Verification items for this drawing (mm, ordinates from the low corner). A direction names the side the tool comes from. Coordinates: 2 decimals unless noted, no trailing zeros. Order: outer loops, then holes, each group sorted by start corner. A loop starts at its lowest first (then second) coordinate and runs counter-clockwise, first axis right, second up.
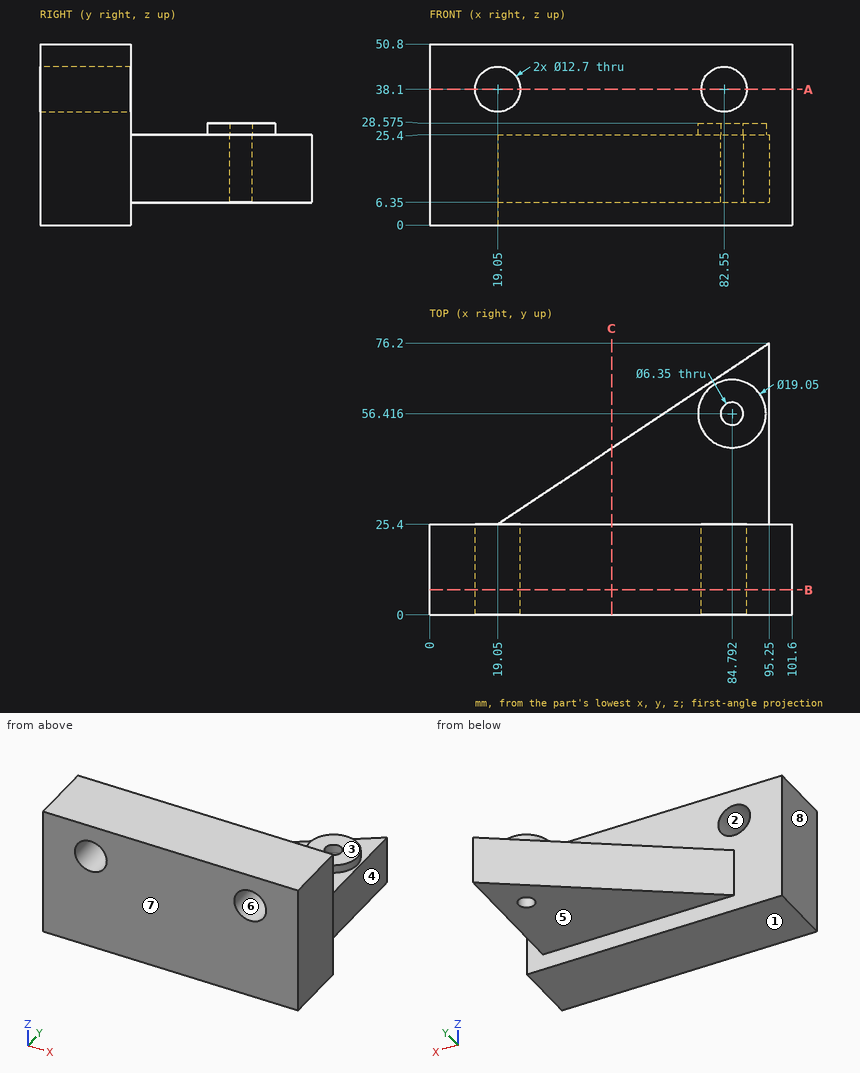
(1) Cross-section at B-B (y = 7). Enter the section's corners in (x, z), and give its area (3 significant figures).
Filled in:
outline: (0, 0) - (101.6, 0) - (101.6, 50.8) - (0, 50.8) - close; hole circle Ø12.7 at (19.05, 38.1); hole circle Ø12.7 at (82.55, 38.1)
area: 4,910 mm2
(2) Cross-section at A-A (z = 38.1). Enter the section's corners in (x, y).
Filled in:
outline: (0, 0) - (12.7, 0) - (12.7, 25.4) - (0, 25.4) - close; (25.4, 0) - (76.2, 0) - (76.2, 25.4) - (25.4, 25.4) - close; (88.9, 0) - (101.6, 0) - (101.6, 25.4) - (88.9, 25.4) - close
(3) Cross-section at C-C (x = 51). Enter the section's corners in (y, z).
Filled in:
outline: (0, 0) - (25.4, 0) - (25.4, 6.35) - (46.7, 6.35) - (46.7, 25.4) - (25.4, 25.4) - (25.4, 50.8) - (0, 50.8) - close
(4) Go/stop test with flat-tipped pins: P1, Ø2, axis at x = 31, z = 30.5, coming from the +Y side; P2, Ø8.5, axis at x = 84.79, y = 56.42, coming from the +Z side (3 decimals); P3, Ø15, axis at x = 67, y = 54.5, coming from the +Z side. Record where each tip stops, or that it passes through.
Filled in:
P1: stops at y = 25.4
P2: stops at z = 28.575
P3: stops at z = 25.4
(5) Tool access check on the marked faces 1, 2, 3, 4 and 5. Record the directions out of +Z, -Z, +X, -X, +Y, -Y that give a thin tool (end or side, any length) a straight path to the whole face; none if there is none.
Filled in:
face 1: -Z, +X, -X, +Y, -Y
face 2: +Y, -Y
face 3: +Z, +X, -X, +Y
face 4: +Z, -Z, +X, +Y
face 5: -Z, +X, -X, +Y
(6) Release check for a two-part mould opening along X. For the marked faces 6, 7 and 8 record: +X half, -X half, draft (parallel to the pull), parting line (faces both ways), or undercut.
Filled in:
face 6: undercut
face 7: draft
face 8: -X half
(7) Thickness scan on probe 1 along X at (y, z) = (18, 38); probe 2 along X at (y, z) = (23.5, 36); probe 3 along Y at (x, z) = (19, 29). Record the ranges inside material, lowest first.
Filled in:
probe 1: x = 0 to 12.7, 25.4 to 76.2, 88.9 to 101.6
probe 2: x = 0 to 13.06, 25.04 to 76.56, 88.54 to 101.6
probe 3: y = 0 to 25.4
